Geometry: see drawing. Coordinates: mm, zero at the bounding-box minimum. A direction names the side the tool comes from. Round coordinates to 2 decimals unless told otherwise and drop trailing zeros. Write each loop counter-clockwise with the first axis right and the second up, starting at its lowest first coordinate (ties: lowest second). Pieces come first, ordered by that corner, then holes.
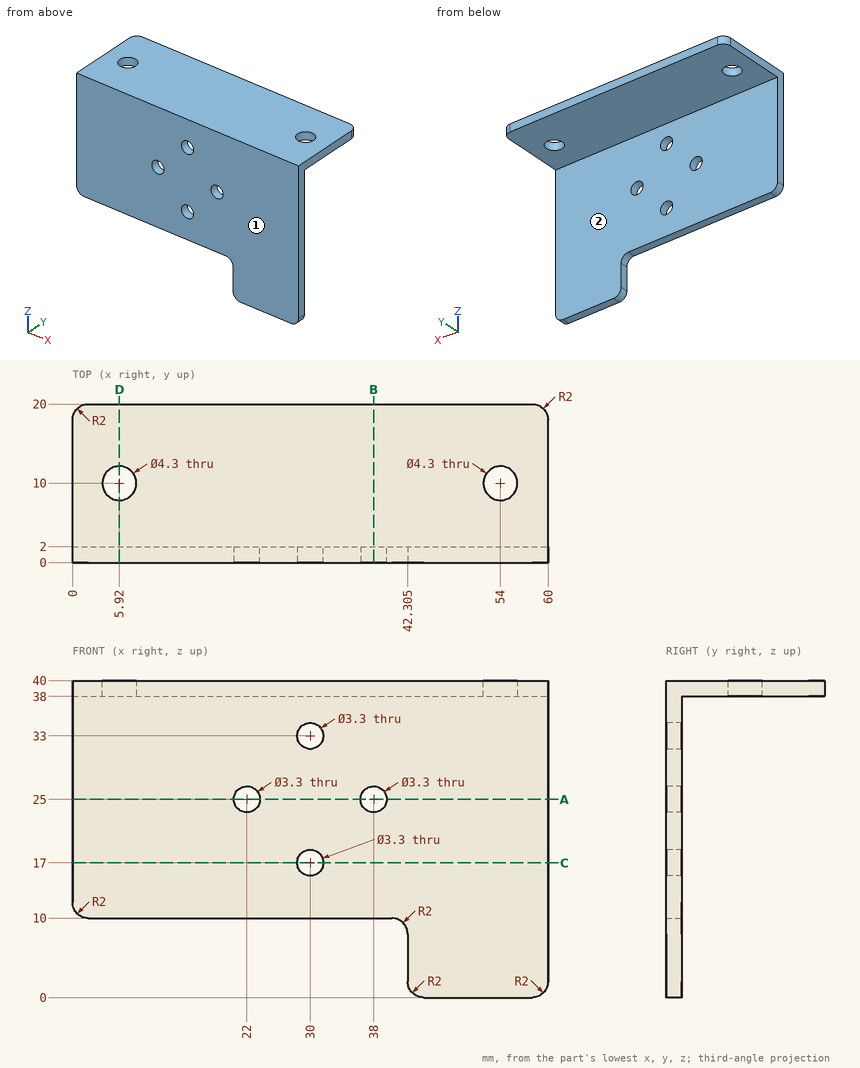
1) Material intervals for line 1 (Z direction, x = 30, y = 0.4); line 2 (Z direction, x = 38, y = 1.3); line 3 (X direction, y = 1.45, z = 17), sorted ascending.
Taken from the geometry:
line 1: z = 10 to 15.35, 18.65 to 31.35, 34.65 to 40
line 2: z = 10 to 23.35, 26.65 to 40
line 3: x = 0 to 28.35, 31.65 to 60
2) Section query D-D on x = 5.92. Return the cut outline in (y, z).
Taken from the geometry:
outline: (0, 10) - (2, 10) - (2, 38) - (7.85, 38) - (7.85, 40) - (0, 40) - close; (12.15, 38) - (20, 38) - (20, 40) - (12.15, 40) - close
3) Section query A-A on z = 25. Return the cut outline in (x, y).
Taken from the geometry:
outline: (0, 0) - (20.35, 0) - (20.35, 2) - (0, 2) - close; (23.65, 0) - (36.35, 0) - (36.35, 2) - (23.65, 2) - close; (39.65, 0) - (60, 0) - (60, 2) - (39.65, 2) - close
4) Contact query for flat-ended pins moving along their axis: P1, Ø1.6, axis at x = 13.5, y = 0.5, coming from the -Z side; P2, Ø19, axis at x = 38, z = 16.5, coming from the +Y side; P3, Ø4, axis at x = 48, y = 14, coming from the -Z side. Output: stop coordinate, or through.
Taken from the geometry:
P1: stops at z = 10
P2: stops at y = 2
P3: stops at z = 38
5) Reachability of the marked faces 1 and 2 from +Z, -Z, +X, -X, +Y, -Y: full face, straight path, thin tool, end or side. Return the list, or none.
Taken from the geometry:
face 1: +Z, -Z, +X, -X, -Y
face 2: -Z, +X, -X, +Y
6) Section query C-C on z = 17. Return the cut outline in (x, y), then the cut area to 3 significant figures.
Taken from the geometry:
outline: (0, 0) - (28.35, 0) - (28.35, 2) - (0, 2) - close; (31.65, 0) - (60, 0) - (60, 2) - (31.65, 2) - close
area: 113 mm2
7) Section query B-B on x = 38. Return the cut outline in (y, z).
Taken from the geometry:
outline: (0, 10) - (2, 10) - (2, 23.35) - (0, 23.35) - close; (0, 26.65) - (2, 26.65) - (2, 38) - (20, 38) - (20, 40) - (0, 40) - close
